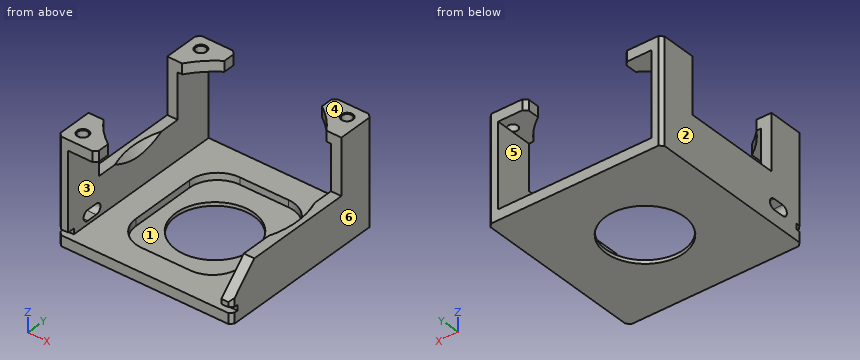
from build123d import *

# Parameters (mm, degrees)
SKETCH_1_W                   = 50
SKETCH_1_H                   = 30
SKETCH_1_W_2                 = 44
SKETCH_1_H_2                 = 24
EXTRUDE_1_DEPTH              = 50
CUT_EXTRUDE_START            = -14
CUT_EXTRUDE_1_DEPTH          = 17
SKETCH_3_R                   = 11.25
CUT_EXTRUDE_2_DEPTH          = 4
HOLE_WIZARD_4_40_D           = 2.8448
HOLE_WIZARD_4_40_DEPTH       = 3
HOLE_WIZARD_4_40_CSINK_D     = 3.3528
HOLE_WIZARD_4_40_CSINK_ANGLE = 110
SKETCH_10_W                  = 1.6
SKETCH_10_H                  = 2
CUT_EXTRUDE_4_DEPTH          = 51
CUT_EXTRUDE_3_DEPTH          = 2
CHAMFER_1_SIZE               = 8
CHAMFER_2_SIZE               = 1
CUT_EXTRUDE_5_REACH          = 52


with BuildPart() as part:
    # Эскиз1 → Бобышка-Вытянуть1 (new body)
    with BuildSketch(Plane(origin=(0, 0, 0), x_dir=(1, 0, 0), z_dir=(0, 1, 0))):
        Rectangle(SKETCH_1_W, SKETCH_1_H)
        Rectangle(SKETCH_1_W_2, SKETCH_1_H_2, mode=Mode.SUBTRACT)
    extrude(amount=EXTRUDE_1_DEPTH)

    # Эскиз2 → Вырез-Вытянуть1 (cut, through all)
    with BuildSketch(Plane(origin=(0, 0, -15), x_dir=(-1, 0, 0), z_dir=(0, 0, -1)).offset(CUT_EXTRUDE_START)):
        with BuildLine():
            ThreePointArc((-14, 45.712315177), (-17.67766953, 42.67766953), (-20.712315177, 39))
            Line((-20.712315177, 39), (-25, 39))
            Line((-25, 39), (-25, 11))
            Line((-25, 11), (-20.712315177, 11))
            ThreePointArc((-20.712315177, 11), (-17.67766953, 7.32233047), (-14, 4.287684823))
            Line((-14, 4.287684823), (-14, 0))
            Line((-14, 0), (14, 0))
            Line((14, 0), (14, 4.287684823))
            ThreePointArc((14, 4.287684823), (17.67766953, 7.32233047), (20.712315177, 11))
            Line((20.712315177, 11), (25, 11))
            Line((25, 11), (25, 39))
            Line((25, 39), (20.712315177, 39))
            ThreePointArc((20.712315177, 39), (17.67766953, 42.67766953), (14, 45.712315177))
            Line((14, 45.712315177), (14, 50))
            Line((14, 50), (-14, 50))
            Line((-14, 50), (-14, 45.712315177))
        make_face()
        with BuildLine():
            Line((-20.712315177, 11), (-25, 11))
            Line((-25, 11), (-25, 0))
            Line((-25, 0), (-14, 0))
            Line((-14, 0), (-14, 4.287684823))
            ThreePointArc((-14, 4.287684823), (-17.67766953, 7.32233047), (-20.712315177, 11))
        make_face()
    extrude(amount=-CUT_EXTRUDE_1_DEPTH, mode=Mode.SUBTRACT)

    # Эскиз3 → Вырез-Вытянуть2 (cut, through all)
    with BuildSketch(Plane.XY.offset(-12)):
        with Locations((0, 25)):
            Circle(SKETCH_3_R)
    extrude(amount=-CUT_EXTRUDE_2_DEPTH, mode=Mode.SUBTRACT)

    # Эскиз6 → Вырез-Повернуть1 (revolve, cut)
    with BuildSketch(Plane(origin=(0, 25, 0), x_dir=(-1, 0, 0), z_dir=(0, 1, 0))):
        Polygon((-22, -3.309797446), (-22, -1), (-23.5, -1), align=None)
    revolve(axis=Axis((0, 25, -15), (0, 0, 1)), mode=Mode.SUBTRACT)

    # Отверстие #4-40
    with Locations(Plane.XY.offset(15)):
        with Locations((-21, 46), (21, 46), (-21, 4)):
            CounterSinkHole(HOLE_WIZARD_4_40_D / 2, HOLE_WIZARD_4_40_CSINK_D / 2, depth=HOLE_WIZARD_4_40_DEPTH, counter_sink_angle=HOLE_WIZARD_4_40_CSINK_ANGLE)

    # Эскиз10 → Вырез-Вытянуть4 (cut, through all)
    with BuildSketch(Plane.ZY.offset(25)):
        with Locations((-11.2, 1)):
            Rectangle(SKETCH_10_W, SKETCH_10_H)
    extrude(amount=-CUT_EXTRUDE_4_DEPTH, mode=Mode.SUBTRACT)

    # Эскиз9 → Вырез-Вытянуть3 (cut)
    with BuildSketch(Plane.XY.offset(-12)):
        with BuildLine():
            Line((-7, 7.5), (7, 7.5))
            ThreePointArc((7, 7.5), (12.656854249, 9.843145751), (15, 15.5))
            Line((15, 15.5), (15, 34.5))
            ThreePointArc((15, 34.5), (12.656854249, 40.156854249), (7, 42.5))
            Line((7, 42.5), (-7, 42.5))
            ThreePointArc((-7, 42.5), (-12.656854249, 40.156854249), (-15, 34.5))
            Line((-15, 34.5), (-15, 15.5))
            ThreePointArc((-15, 15.5), (-12.656854249, 9.843145751), (-7, 7.5))
        make_face()
    extrude(amount=-CUT_EXTRUDE_3_DEPTH, mode=Mode.SUBTRACT)

    # Фаска1
    chamfer_1_edges = [part.edges().sort_by_distance(p)[0] for p in [
        (23.5, 0, -1),
    ]]
    chamfer(chamfer_1_edges, length=CHAMFER_1_SIZE)

    # Фаска2
    chamfer_2_edges = [part.edges().sort_by_distance(p)[0] for p in [
        (-25, 50, 0),
        (25, 0, -13.5),
        (-25, 0, 2.3),
        (25, 0, -9.7),
        (25, 50, 0),
        (-25, 0, -13.5),
        (14, 50, 13.5),
        (-14, 50, 13.5),
        (-14, 0, 13.5),
    ]]
    chamfer(chamfer_2_edges, length=CHAMFER_2_SIZE)

    # Эскиз11 → Вырез-Вытянуть5 (cut, up to next)
    with BuildSketch(Plane.ZY.offset(25), mode=Mode.PRIVATE) as cut_extrude_5_sk1:
        with BuildLine():
            Line((-8, 10), (-8, 7))
            ThreePointArc((-8, 7), (-9.5, 5.5), (-11, 7))
            Line((-11, 7), (-11, 10))
            ThreePointArc((-11, 10), (-9.5, 11.5), (-8, 10))
        make_face()
    cut_extrude_5_tool1 = extrude(cut_extrude_5_sk1.sketch, amount=-CUT_EXTRUDE_5_REACH, mode=Mode.PRIVATE) & part.part
    add(cut_extrude_5_tool1.solids().sort_by_distance((-25, 8.5, -9.5))[0], mode=Mode.SUBTRACT)


solid = part.part
Can you work these out from the model? Positions are in its coordinate system, mm. Face numbers are marked on the shaded views. A direction names the side the tool comes from. Coordinates: 2 decimals unless noted, no trailing zeros. Write each loop counter-clockwise with the first axis right and the second up, starting at its lowest first coordinate (ties: lowest second). Pieces come first, ordered by that corner, then holes. Notation, with made-up numbers: (30, 61) -> (36, 61) arc R35 ccw to (36, 94) -> close; hole circle Ø10 at (54, -32.5). An arc over 180 degrees is marked (long way). Write item = value, one per line.
(1) For pin 1 (2.5 mm diameter, centred on x = 21, y = 46, fed in from +Z); pin 2 (0.5 mm diameter, centred on x = -24, z = -11, fed in from -Y); pin 3 (1.5 mm diameter, centred on x = 3.5, y = 14.5, fed in from +Z); pin 4 (10 mm diameter, centred on x = -19, z = -1.5, fed in from +Y), each with a flat end and sliding along its axis, tell me the tip position at first contact or that it passes through.
Verdict:
pin_1 = 12
pin_2 = 2
pin_3 = -14
pin_4 = 50
(2) If I drill on probe 1 along Z at (x, y) = (-21.5, 8.5); probe 2 along Y at (x, z) = (-21, 13.25); probe 3 along X at (y, z) = (46, 12.8), over which ranges is the centre line in solid material (lowest first)?
Verdict:
probe_1 = -15 to -12, 12 to 15
probe_2 = 0 to 2.58, 5.42 to 11, 39 to 44.58, 47.42 to 50
probe_3 = -25 to -22.42, -19.58 to -14, 14 to 19.58, 22.42 to 25
(3) Imagine slicing it at C-C (y = 25). Please give me the cut outline in (x, z), and give its area (3 significant figures).
Verdict:
outline = (-25, -15) -> (-11.25, -15) -> (-11.25, -14) -> (-15, -14) -> (-15, -12) -> (-22, -12) -> (-22, -3.31) -> (-23.5, -1) -> (-25, -1) -> close; (11.25, -15) -> (25, -15) -> (25, -1) -> (23.5, -1) -> (22, -3.31) -> (22, -12) -> (15, -12) -> (15, -14) -> (11.25, -14) -> close
area = 130 mm^2
(4) Thinking about a two-plate mould opening in Z: for the marked faces 4, 5 and 6, which applies, +Z half, -Z half, draft (parallel to the pull), parting line (faces both ways), or undercut?
Verdict:
face_4 = +Z half
face_5 = undercut
face_6 = draft
(5) Imagine slicing it at D-D (x = -16.5). Please give me the cut outline in (y, z).
Verdict:
outline = (0, -15) -> (50, -15) -> (50, -12) -> (0, -12) -> close; (0, 12) -> (6.22, 12) -> (6.22, 15) -> (0, 15) -> close; (43.78, 12) -> (50, 12) -> (50, 15) -> (43.78, 15) -> close
(6) Imagine slicing it at B-B (z = 9.5). Please give me the cut outline in (x, y), and give its area (3 significant figures).
Verdict:
outline = (-25, 1) -> (-24, 0) -> (-22, 0) -> (-22, 11) -> (-25, 11) -> close; (-25, 39) -> (-22, 39) -> (-22, 50) -> (-24, 50) -> (-25, 49) -> close; (22, 39) -> (25, 39) -> (25, 49) -> (24, 50) -> (22, 50) -> close
area = 97.5 mm^2
(7) On a 3-axis mill with a long thin cutter (end or side, diameter ignored), from which of +Z, -Z, +X, -X, +Y, -Y can I reach the whole of each face in a straight line? I mean the marked faces 1, 2 and 3. Say none if no direction works.
Verdict:
face_1 = +Z
face_2 = +Z, -Z, -X, +Y, -Y
face_3 = +Y, -Y
(8) Imagine slicing it at A-A (x = 0). Please give me the cut outline in (y, z), and give its area (3 significant figures).
Verdict:
outline = (0, -15) -> (13.75, -15) -> (13.75, -14) -> (7.5, -14) -> (7.5, -12) -> (0, -12) -> close; (36.25, -15) -> (50, -15) -> (50, -12) -> (42.5, -12) -> (42.5, -14) -> (36.25, -14) -> close
area = 57.5 mm^2
